from build123d import *

# Parameters (mm, degrees)
SKETCH1_W           = 45
SKETCH1_H           = 50
BOSS_EXTRUDE1_DEPTH = 3
SKETCH4_W           = 12.5
SKETCH4_H           = 40.003655499
SKETCH4_H_2         = 40
SKETCH4_W_2         = 10
SKETCH4_H_3         = 4
CUT_EXTRUDE1_DEPTH  = 3


with BuildPart() as part:
    # Sketch1 → Boss-Extrude1 (new body)
    with BuildSketch(Plane(origin=(0, 0, 0), x_dir=(1, 0, 0), z_dir=(0, 1, 0))):
        Rectangle(SKETCH1_W, SKETCH1_H)
    extrude(amount=BOSS_EXTRUDE1_DEPTH)

    # Sketch4 → Cut-Extrude1 (cut)
    with BuildSketch(Plane(origin=(0, 3, 0), x_dir=(1, 0, 0), z_dir=(0, 1, 0))):
        with Locations((-16.25, 4.99817225)):
            Rectangle(SKETCH4_W, SKETCH4_H)
        with Locations((16.25, 5)):
            Rectangle(SKETCH4_W, SKETCH4_H_2)
        with Locations((0, -6)):
            Rectangle(SKETCH4_W_2, SKETCH4_H_3)
    extrude(amount=-CUT_EXTRUDE1_DEPTH, mode=Mode.SUBTRACT)


solid = part.part
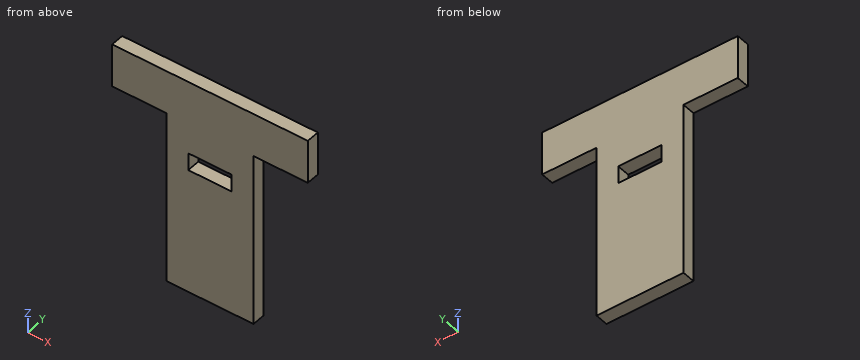
Here's how the part is built. I have some questions about the finished solid (model axes, mm). Give positions to 0.01 mm unless a question says otherwise; leave off trailing zeros. Loops run counter-clockwise (first coordinate to the right, second up) from the corner with the lowest first, then second, coordinate; pieces in that order, holes last. Notation, with made-up numbers: (85, 32) -> (125, 32) arc R9 ccw to (125, 42) -> close; hole circle Ø7 at (86, 70). An arc over 180 degrees is marked (long way). Answer as a JSON object with one key per item and string values. Group by question number.
Item 1: Imagine slicing it at B-B on y = 1.35. Write out the boundary of the cut face in (x, z).
Item 2: Will these pins go through, and if not, where does the flat tip stop? pin 1 (1.5 mm diameter, centred on y = 1, z = 5.5, fed in from -X); pin 2 (1.5 mm diameter, centred on x = -16.5, y = 2, fed in from -Z); pin 3 (1.5 mm diameter, centred on y = 2, z = 6, fed in from +X).
Item 3: Imagine slicing it at D-D on x = -15.5. Write out the boundary of the cut face in (y, z), then the cut area to 3 significant figures.
Item 4: Imagine slicing it at C-C on z = -12. Write out the boundary of the cut face in (x, y), then the cut area to 3 significant figures.
Item 5: Imagine slicing it at A-A on x = -0.5. Write out the boundary of the cut face in (y, z).
Item 6: I need wall thicknesses on L1, parallel to X at y = 1.85, z = 6; L2, parallel to Z at x = 4.5, y = 2.3; L3, parallel to X at y = 2.5, z = -17. Which ranges of each line are inside material? Lowest first, please.
Answer list:
{
 "1": {"outline": "(-22.5, 15) -> (-10, 15) -> (-10, -25) -> (10, -25) -> (10, 15) -> (22.5, 15) -> (22.5, 25) -> (-22.5, 25) -> close; hole (-5, 4) -> (5, 4) -> (5, 8) -> (-5, 8) -> close"},
 "2": {"pin 1": "stops at x = -10", "pin 2": "stops at z = 15", "pin 3": "stops at x = 10"},
 "3": {"outline": "(0, 15) -> (3, 15) -> (3, 25) -> (0, 25) -> close", "area": "30.0 mm2"},
 "4": {"outline": "(-10, 0) -> (10, 0) -> (10, 3) -> (-10, 3) -> close", "area": "60.0 mm2"},
 "5": {"outline": "(0, -25) -> (3, -25) -> (3, 4) -> (0, 4) -> close; (0, 8) -> (3, 8) -> (3, 25) -> (0, 25) -> close"},
 "6": {"L1": "x = -10 to -5, 5 to 10", "L2": "z = -25 to 4, 8 to 25", "L3": "x = -10 to 10"}
}
